Autodesk Inventor part; units mm, degrees
ref_plane "YZ Plane" through (0, 0, 0) normal (1, 0, 0) x (0, 1, 0)
ref_plane "XZ Plane" through (0, 0, 0) normal (0, 1, 0) x (-1, 0, 0)
ref_plane "XY Plane" through (0, 0, 0) normal (0, 0, 1) x (1, 0, 0)
sketch "Sketch1" plane through (0, 0, 0) normal (0, 1, 0) x (-1, 0, 0)
  circle A0 centre (0, 0) radius 19.25
  circle A1 centre (23.57, -23.57) radius 2.6
  circle A2 centre (23.57, 23.57) radius 2.6
  circle A3 centre (-23.57, 23.57) radius 2.6
  circle A4 centre (-23.57, -23.57) radius 2.6
  circle A5 centre (23.57, 23.57) radius 5.775 construction
  circle A6 centre (23.57, -23.57) radius 5.775 construction
  circle A7 centre (-23.57, -23.57) radius 5.775 construction
  circle A8 centre (-23.57, 23.57) radius 5.775 construction
  line L0 (29.345, 23.57) -> (29.345, -23.57)
  line L1 (23.57, -29.345) -> (-23.57, -29.345)
  line L2 (-29.345, -23.57) -> (-29.345, 23.57)
  line L3 (-23.57, 29.345) -> (23.57, 29.345)
  arc A9 (-29.345, -23.57) -> (-23.57, -29.345) centre (-23.57, -23.57) ccw
  arc A10 (-23.57, 29.345) -> (-29.345, 23.57) centre (-23.57, 23.57) ccw
  arc A11 (23.57, -29.345) -> (29.345, -23.57) centre (23.57, -23.57) ccw
  arc A12 (29.345, 23.57) -> (23.57, 29.345) centre (23.57, 23.57) ccw
  dimension "d0" = 38.5
  dimension "d1" = 5.2
  dimension "d2" = 23.57
  dimension "d3" = 23.57
  dimension "d4" = 23.57
  dimension "d5" = 23.57
  dimension "d6" = 3.175
extrude "Extrusion1" add sketch "Sketch1" along normal blind 1.6625
properties part number "CNC-004-Nema23Shim" material "ABS Plastic"
Can you work these out from the model? Positions are in its coordinate system, mm. Coordinates: 2 decimals unless noted, no trailing zeros. Loops run counter-clockwise (first coordinate to the right, second up) from the corner with the lowest first, then second, coordinate; pieces in that order, holes last. Notation, with made-up numbers: (-15, -17.75) - (1, -17.75) arc R22 ccw to (1, 10.25) - close; hole circle Ø10 at (-37.75, 30). An arc over 180 degrees is marked (long way). Put each result on its own line as item: value. Start each with the question number.
Item 1: If we mould it in two halves opening along X, with no side actions, what happens to faces 1 (the face through (-27.698, 0.82, -27.608)), 2 (the face through (27.698, 0.82, 27.608)), 3 (the face through (15.28, 0.82, 11.71))? For each: +X half, -X half, draft (parallel to the pull), parting line (faces both ways), or undercut.
Item 2: Suppose I cut it at C-C (y = 0.7). Please give me the cut outline in (x, z) (3 decimals).
Item 3: If I drill on line 1 along Z through (x, y) = (-23.57, 0.55) (3 decimals); line 2 along Z through (x, y) = (0, 1.35) (3 decimals); line 3 along X through (y, z) = (1.1, -24), over which ranges is the centre line in solid material (lowest first)?
Item 4: For pin 1 (8.5 mm diameter, centred on x = 23.57, z = -23.57, fed in from +Y), with a flat end and sliding along its axis, tell me the tip position at first contact or that it passes through.
Here are the results:
1. face 1: -X half
1. face 2: +X half
1. face 3: undercut
2. outline: (-29.345, -23.57) arc R5.775 ccw to (-23.57, -29.345) - (23.57, -29.345) arc R5.775 ccw to (29.345, -23.57) - (29.345, 23.57) arc R5.775 ccw to (23.57, 29.345) - (-23.57, 29.345) arc R5.775 ccw to (-29.345, 23.57) - close; hole circle Ø5.2 at (-23.57, -23.57); hole circle Ø5.2 at (-23.57, 23.57); hole circle Ø38.5 at (0, 0); hole circle Ø5.2 at (23.57, -23.57); hole circle Ø5.2 at (23.57, 23.57)
3. line 1: -29.345 to -26.17, -20.97 to 20.97, 26.17 to 29.345
3. line 2: -29.345 to -19.25, 19.25 to 29.345
3. line 3: -29.33 to -26.13, -21.01 to 21.01, 26.13 to 29.33
4. pin 1: y = 1.66
